Can you work these out from the model? Positions are in its coordinate system, mm. Face numbers are marked on the shaded views. A direction names the side the tool comes from. Give positions to 0.01 mm unless a question says otherwise; leave off trailing zeros. Write each loop counter-clockwise with the first axis right and the second up, starting at its lowest first coordinate (ties: lowest second). Pieces come first, ordered by that corner, then holes.
Autodesk Inventor part; units mm, degrees
ref_plane "Work Plane1" through (0, 10, 0) normal (0, 1, 0) x (1, 0, 0)
ref_plane "YZ Plane" through (0, 0, 0) normal (1, 0, 0) x (0, 1, 0)
ref_plane "XZ Plane" through (0, 0, 0) normal (0, 1, 0) x (-1, 0, 0)
sketch "Sketch1" plane through (0, 0, 0) normal (1, 0, 0) x (0, 1, 0)
  circle A0 centre (0, 0) radius 6
  circle A1 centre (0, 0) radius 10
  line L0 (0, 10) -> (-10, 10)
  line L1 (-10, 10) -> (-10, -10)
  line L2 (-10, -10) -> (0, -10)
  line L3 (-10, -10) -> (-7, -10)
  line L4 (-7, -10) -> (-7, -25)
  line L5 (-7, -25) -> (-10, -25)
  line L6 (-10, -25) -> (-10, -10)
  line L7 (-10, 10) -> (-7, 10)
  line L8 (-7, 10) -> (-7, 25)
  line L9 (-7, 25) -> (-10, 25)
  line L10 (-10, 25) -> (-10, 10)
  dimension "d0" = 12
  dimension "d1" = 20
  dimension "d2" = 3
  dimension "d3" = 15
  dimension "d4" = 3
  dimension "d5" = 15
extrude "Extrusion1" add sketch "Sketch1" along normal blind 30
sketch "Sketch2" plane through (0, -7, 25) normal (0, 1, 0) x (1, 0, 0)
  line L0 (0, 0) -> (30, 0)
  line L1 (0, 0) -> (15, 0)
  line L2 (15, 0) -> (15, 7.5)
  line L3 (15, 7.5) -> (0, 7.5)
  line L4 (0, 7.5) -> (0, 0)
  line L5 (30, 0) -> (30, 50)
  line L6 (30, 50) -> (15, 50)
  line L7 (15, 50) -> (15, 42.5)
  line L8 (15, 42.5) -> (30, 42.5)
  line L9 (30, 42.5) -> (30, 50)
  circle A0 centre (15, 7.5) radius 3
  circle A1 centre (15, 42.5) radius 3
  point P0 (0, 25)
  dimension "d8" = 15
  dimension "d9" = 7.5
  dimension "d10" = 15
  dimension "d11" = 7.5
  dimension "d12" = 6
  dimension "d13" = 6
ref_plane "Work Plane1" through (0, 10, 0) normal (0, 1, 0) x (1, 0, 0)
sketch "Sketch3" plane through (0, 10, 0) normal (0, 1, 0) x (1, 0, 0)
  line L0 (0, 0) -> (15, 0)
  circle A0 centre (15, 0) radius 2
  dimension "d14" = 15
  dimension "d15" = 4
hole "Hole1" at (15, 10, 0) direction (0, -1, 0) diameter 4 depth 8 tip angle 118
thread "Thread1"
hole "Hole2" at (15, -7, 17.5) at (15, -7, -17.5) direction (0, -1, 0) diameter 6 end through all
properties part number "base_axis_static_12mm" material "PET Plastic"
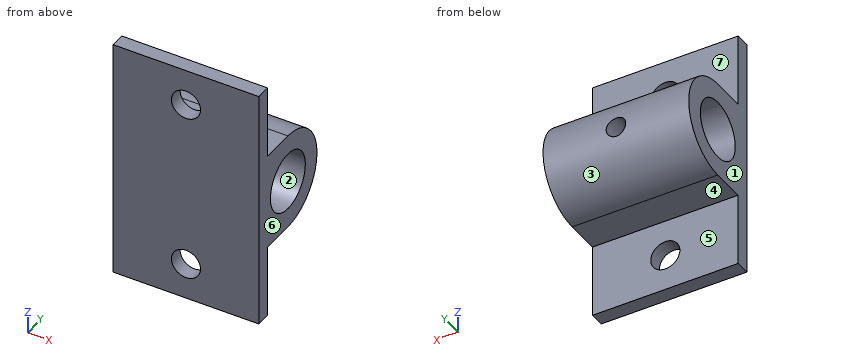
(1) Imagine slicing it at A-A, the plane z = 0. Write out the boundary of the cut face in (x, y).
Returned:
outline: (0, -10) - (30, -10) - (30, -6) - (0, -6) - close; (0, 6) - (13, 6) - (13, 10) - (0, 10) - close; (17, 6) - (30, 6) - (30, 10) - (17, 10) - close
(2) For the marked faces 5, 6 and 7, which set-ups out of +Z, -Z, +X, -X, +Y, -Y let a thin tool reach every point of the face, with its end or its side?
Returned:
face 5: -Z, +X, -X, +Y
face 6: +Z, -Z, +X, +Y, -Y
face 7: +Z, +X, -X, +Y
(3) Will these pins go through, and if not, where does the flat tip stop? P1, Ø12, axis at x = 11, z = 18.5, coming from the +Y side; P2, Ø5.5, axis at x = 17.5, y = -2, coming from the -Z side; P3, Ø2.5, axis at x = 15, z = 0, coming from the +Y side.
Returned:
P1: stops at y = -7
P2: stops at z = -10
P3: stops at y = -5.87
(4) If I drill on L1, parallel to Z at x = 15, y = -9.15; L2, parallel to Z at x = 2.5, y = 0; L3, parallel to Z at x = 17, y = -8, over which ranges is the centre line in solid material (lowest first)?
Returned:
L1: z = -25 to -20.5, -14.5 to 14.5, 20.5 to 25
L2: z = -10 to -6, 6 to 10
L3: z = -25 to -19.74, -15.26 to 15.26, 19.74 to 25
(5) If we mould it in two halves opening along Z, with no side actions, what happens to the marked faces 1, 2, 3 and 4? For each: +Z half, -Z half, draft (parallel to the pull), parting line (faces both ways), or undercut.
Returned:
face 1: draft
face 2: undercut
face 3: parting line
face 4: -Z half
(6) Imagine slicing it at D-D, the plane x = 15. Write out the boundary of the cut face in (y, z).
Returned:
outline: (-10, -25) - (-7, -25) - (-7, -20.5) - (-10, -20.5) - close; (-10, -14.5) - (-7, -14.5) - (-7, -10) - (0, -10) arc R10 ccw to (9.8, -2) - (5.66, -2) arc R6 cw (long way) to (5.66, 2) - (9.8, 2) arc R10 ccw to (0, 10) - (-7, 10) - (-7, 14.5) - (-10, 14.5) - close; (-10, 20.5) - (-7, 20.5) - (-7, 25) - (-10, 25) - close
(7) Imagine slicing it at C-C, the plane x = 10. Write out the boundary of the cut face in (y, z).
Returned:
outline: (-10, -25) - (-7, -25) - (-7, -10) - (0, -10) arc R10 ccw to (0, 10) - (-7, 10) - (-7, 25) - (-10, 25) - close; hole circle Ø12 at (0, 0)
(8) Imagine slicing it at B-B, the plane y = 3.5. Write out the boundary of the cut face in (x, z), plus the area to 3 significant figures.
Returned:
outline: (0, -9.37) - (30, -9.37) - (30, -4.87) - (0, -4.87) - close; (0, 4.87) - (30, 4.87) - (30, 9.37) - (0, 9.37) - close
area: 270 mm2
